from build123d import *

# Parameters (mm, degrees)
EXTRUDE_1_DEPTH     = 12
EXTRUDE_2_DEPTH     = 1
SKETCH_2_W          = 8
SKETCH_2_H          = 8
SKETCH_2_R          = 3.2
EXTRUDE_3_DEPTH     = 10
CUT_EXTRUDE_2_REACH = 35.151
SKETCH_2_2_R        = 3.2
SKETCH_2_4_W        = 2
SKETCH_2_4_H        = 8
EXTRUDE_4_DEPTH     = 6
CHAMFER_1_SIZE      = 2
EXTRUDE_START       = -19.6
SKETCH_2_5_W        = 2
SKETCH_2_5_H        = 8
EXTRUDE_5_DEPTH     = 2
CHAMFER_2_SIZE      = 2
FILLET_1_R          = 5


with BuildPart() as part:
    # 草图1 → 凸台-拉伸1 (new body)
    with BuildSketch(Plane.XY):
        Polygon((-19.95, -7.8), (7.8, -7.8), (7.8, 7.8), (-19.95, 7.8), (-19.95, 11.8), (11.8, 11.8), (11.8, -11.8), (-19.95, -11.8), align=None)
        with BuildLine():
            Line((-5.15, 7.8), (-7.95, 7.8))
            Line((-7.95, 7.8), (-7.95, 5.8))
            Line((-7.95, 5.8), (-7.719046516, 5.8))
            ThreePointArc((-7.719046516, 5.8), (-6.77788206, 7.241052367), (-5.15, 7.8))
        make_face()
        with BuildLine():
            Line((-7.95, -5.8), (-7.95, -7.8))
            Line((-7.95, -7.8), (-5.15, -7.8))
            ThreePointArc((-5.15, -7.8), (-6.77788206, -7.241052367), (-7.719046516, -5.8))
            Line((-7.719046516, -5.8), (-7.95, -5.8))
        make_face()
        with BuildLine():
            ThreePointArc((7.8, -5.15), (7.02383297, -7.02383297), (5.15, -7.8))
            Line((5.15, -7.8), (7.8, -7.8))
            Line((7.8, -7.8), (7.8, -5.15))
        make_face()
        with BuildLine():
            ThreePointArc((5.15, 7.8), (7.02383297, 7.02383297), (7.8, 5.15))
            Line((7.8, 5.15), (7.8, 7.8))
            Line((7.8, 7.8), (5.15, 7.8))
        make_face()
    extrude(amount=-EXTRUDE_1_DEPTH)

    # 草图1<3> → 凸台-拉伸2 (add)
    with BuildSketch(Plane.XY):
        Polygon((-7.95, -7.8), (-19.95, -7.8), (-19.95, -11.8), (11.8, -11.8), (11.8, 11.8), (-19.95, 11.8), (-19.95, 7.8), (-7.95, 7.8), (-7.95, 5.8), (5.8, 5.8), (5.8, -5.8), (-7.95, -5.8), align=None)
    extrude(amount=EXTRUDE_2_DEPTH)

    # 草图2 → 凸台-拉伸3 (add)
    with BuildSketch(Plane.XZ.offset(11.8)):
        with Locations((-13.95, -6)):
            Rectangle(SKETCH_2_W, SKETCH_2_H)
        with Locations(Location((-13.95, -6, 0), (0, 0, 270))):
            Circle(SKETCH_2_R, mode=Mode.SUBTRACT)
    extrude_3 = extrude(amount=-EXTRUDE_3_DEPTH)

    # 草图2<2> → 切除-拉伸2 (cut, up to next)
    with BuildSketch(Plane.XZ.offset(11.8), mode=Mode.PRIVATE) as cut_extrude_2_sk1:
        with Locations(Location((-13.95, -6, 0), (0, 0, 270))):
            Circle(SKETCH_2_2_R)
    cut_extrude_2_tool1 = extrude(cut_extrude_2_sk1.sketch, amount=-CUT_EXTRUDE_2_REACH, mode=Mode.PRIVATE) & part.part
    cut_extrude_2 = cut_extrude_2_tool1.solids().sort_by_distance((-13.95, -11.8, -6))[0]
    add(cut_extrude_2, mode=Mode.SUBTRACT)

    # 草图2<4> → 凸台-拉伸4 (add)
    with BuildSketch(Plane.XZ.offset(11.8)):
        with Locations((-8.95, -6)):
            Rectangle(SKETCH_2_4_W, SKETCH_2_4_H)
    extrude(amount=-EXTRUDE_4_DEPTH)

    # 倒角1
    chamfer_1_edges = [part.edges().sort_by_distance(p)[0] for p in [
        (-9.95, -5.8, -6),
    ]]
    chamfer(chamfer_1_edges, length=CHAMFER_1_SIZE)

    # 镜向6: 凸台-拉伸3, 切除-拉伸2 across plane
    add(extrude_3.mirror(Plane.ZX))
    add(cut_extrude_2.mirror(Plane.ZX), mode=Mode.SUBTRACT)

    # 草图2<5> → 凸台-拉伸5 (add)
    with BuildSketch(Plane.XZ.offset(11.8).offset(EXTRUDE_START)):
        with Locations((-8.95, -6)):
            Rectangle(SKETCH_2_5_W, SKETCH_2_5_H)
    extrude(amount=EXTRUDE_5_DEPTH)

    # 倒角2
    chamfer_2_edges = [part.edges().sort_by_distance(p)[0] for p in [
        (-9.95, 5.8, -6),
    ]]
    chamfer(chamfer_2_edges, length=CHAMFER_2_SIZE)

    # 圆角1
    fillet_1_edges = [part.edges().sort_by_distance(p)[0] for p in [
        (11.8, 11.8, -5.5),
        (11.8, -11.8, -5.5),
    ]]
    fillet(fillet_1_edges, radius=FILLET_1_R)


solid = part.part
The listing builds one solid part. Answer for the finished solid, in the listing's coordinates (mm). A direction names the side the tool comes from. Give positions to 0.01 mm unless a question says otherwise; leave off trailing zeros. Write each loop counter-clockwise with the first axis right and the second up, starting at its lowest first coordinate (ties: lowest second). Pieces come first, ordered by that corner, then holes. Notation, with made-up numbers: (69, -12) - (91, -12) arc R25 cw to (91, 0) - close; hole circle Ø5 at (-19.75, 81.5). An arc over 180 degrees is marked (long way). One line per question, with ' | ' between items. Start each with the question number.
1. Given P1, Ø2.5, axis at x = -13.5, z = -4.5, coming from the +Y side; P2, Ø1, axis at y = -2.5, z = -8.5, coming from the -X side; P3, Ø2, axis at y = -7, z = -11, coming from the -X side; P4, Ø1, axis at y = 7, z = -1, coming from the -X side, each flat-ended and moving along its own axis, determine where each tip first touches the part or whether it passes through.
2. Section B-B, the plane x = 0.5 is taken. Determine the outline of the cut face in (y, z), then the cut area to 3 significant figures.
3. For faces 5 (the face through (0, 7.8, -6)), 6 (the face through (-15, -7.8, -1)), 7 (the face through (-13, 5, -2)), 8 (the face through (-9.95, -3, -6)), 9 (the face through (-17, 1.8, -4)), determine the directions among +Z, -Z, +X, -X, +Y, -Y from which every point of the face is accessible in a straight line to the end or side of a thin tool.
4. Determine the mould class of faces 1 (the face through (-17.95, -5, -6)), 2 (the face through (7.003, 7.044, -5.916)), 3 (the face through (-13, -5, -2)), 4 (the face through (-6.758, -7.256, -5.916)) for opening direction X: +X half, -X half, draft (parallel to the pull), parting line (faces both ways), or undercut.
5. Section A-A, the plane z = -6 is taken. Count the separate pieces of the cut face and the enclosed holes in it, then the cut area to 3 significant figures.
6. Section C-C, the plane x = -13.95 is taken. Determine the outline of the cut face in (y, z).
7. Section D-D, the plane y = -8.5 is taken. Determine the outline of the cut face in (x, z), then the cut area to 3 significant figures.
8. Straight lines are drawn through the part: line 1 (X direction, y = -4.75, z = -6); line 2 (Y direction, x = -1, z = -1.75); line 3 (X direction, y = 7, z = -6.25). For each, find the intervals that lie inside material, in ascending order.
Result:
1) P1: passes through | P2: stops at x = -17.95 | P3: stops at x = -19.95 | P4: stops at x = -7.95
2) outline: (-11.8, -12) - (-7.8, -12) - (-7.8, 0) - (-5.8, 0) - (-5.8, 1) - (-11.8, 1) - close; (5.8, 0) - (7.8, 0) - (7.8, -12) - (11.8, -12) - (11.8, 1) - (5.8, 1) - close | area: 108 mm2
3) face 5: -Z | face 6: -X | face 7: +Z, -X | face 8: +Z, -Z | face 9: +Z, -Z, -X
4) face 1: -X half | face 2: undercut | face 3: draft | face 4: undercut
5) separate pieces: 3 | enclosed holes: 0 | area: 292 mm2
6) outline: (-11.8, -12) - (-7.8, -12) - (-7.8, -10) - (-1.8, -10) - (-1.8, -9.2) - (-11.8, -9.2) - close; (-11.8, -2.8) - (-1.8, -2.8) - (-1.8, -2) - (-7.8, -2) - (-7.8, 1) - (-11.8, 1) - close; (1.8, -10) - (7.8, -10) - (7.8, -12) - (11.8, -12) - (11.8, -9.2) - (1.8, -9.2) - close; (1.8, -2.8) - (11.8, -2.8) - (11.8, 1) - (7.8, 1) - (7.8, -2) - (1.8, -2) - close
7) outline: (-19.95, -12) - (11.5, -12) - (11.5, 1) - (-19.95, 1) - close; hole circle Ø6.4 at (-13.95, -6) | area: 377 mm2
8) line 1: x = -17.95 to -17.15, -10.75 to -9, 7.8 to 11.8 | line 2: y = -11.8 to -7.8, 7.8 to 11.8 | line 3: x = -17.95 to -17.14, -10.76 to -7.05, 7.05 to 11.8
